Design review of the part built by this model. Coordinates are the model's own, in mm. A direction names the side the tool comes from. Coordinates: 2 decimals unless noted, no trailing zeros. Order: outer loops, then holes, each group sorted by start corner. A loop starts at its lowest first (then second) coordinate and runs counter-clockwise, first axis right, second up. Notation, with made-up numbers: M 80.5,42.5 L 124.5,42.5 A8 cw 124.5,52.5 Z; hole C 0.5,13.5 d6. An arc over 180 degrees is marked long. Answer in a Markdown table with one row per item.
from build123d import *

# Parameters (mm, degrees)
SKETCH_1_R          = 3
SKETCH_1_R_2        = 1.55
EXTRUDE_1_DEPTH     = 30
CUT_EXTRUDE_1_DEPTH = 33.5


with BuildPart() as part:
    # 草图1 → 凸台-拉伸1 (new body)
    with BuildSketch(Plane.XY):
        Polygon((15, 0), (15, 12.5), (0, 12.5), (-15, 12.5), (-15, -24), (15, -24), align=None)
        Circle(SKETCH_1_R, mode=Mode.SUBTRACT)
        with Locations((0, 7)):
            Circle(SKETCH_1_R_2, mode=Mode.SUBTRACT)
        with Locations((7, 0)):
            Circle(SKETCH_1_R_2, mode=Mode.SUBTRACT)
        with Locations((0, -7)):
            Circle(SKETCH_1_R_2, mode=Mode.SUBTRACT)
        with Locations((-7, 0)):
            Circle(SKETCH_1_R_2, mode=Mode.SUBTRACT)
    extrude(amount=EXTRUDE_1_DEPTH)

    # 草图2 → 切除-拉伸1 (cut)
    with BuildSketch(Plane(origin=(0, 12.5, 0), x_dir=(1, 0, 0), z_dir=(0, 1, 0))):
        Polygon((-11.4, -15), (-11.4, -3.6), (0, -3.6), (11.4, -3.6), (11.4, -26.4), (0, -26.4), (-11.4, -26.4), align=None)
    extrude(amount=-CUT_EXTRUDE_1_DEPTH, mode=Mode.SUBTRACT)


solid = part.part
(1) For faces 4 (the cylindrical face through (5.77, -0.94, 28.17)), 5 (the flat face through (0, -4, 3.6)), list the 3-axis set-ups (+Z, -Z, +X, -X, +Y, -Y) from which the entire face can be reached by the end or side of a thin tool; tool diameter is ignored.
Return value:
| item | result |
|---|---|
| face 4 | +Z, -Z |
| face 5 | +Y |
(2) For line 1 along Y through (x, z) = (0, 28.1); line 2 along Z through (x, y) = (9, -18.5); line 3 along Y through (x, z) = (7, 2.5), list the stretches that pass through material, from the lowest coordinate up. Write a range as from..to.
Return value:
| item | result |
|---|---|
| line 1 | y = -24..-8.55, -5.45..-3, 3..5.45, 8.55..12.5 |
| line 2 | z = 0..3.6, 26.4..30 |
| line 3 | y = -24..-1.55, 1.55..12.5 |
(3) Insertion check: pin 1 Ø5.5 at (x, y) = (0, 0) entering from +Z; pin 2 Ø3 at (x, z) = (0, 8) entering from +Y. Each pin has a flat end and moves straight along its axis. Give the tip position at first contact, or say it passes through.
Return value:
| item | result |
|---|---|
| pin 1 | passes through |
| pin 2 | stops at y = -21 |
(4) Add section B-B, the plane x = 7. Give the boundary of the cut face in (y, z), and give its area (3 significant figures).
Return value:
| item | result |
|---|---|
| outline | M -24,0 L -1.55,0 L -1.55,3.6 L -21,3.6 L -21,26.4 L -1.55,26.4 L -1.55,30 L -24,30 Z; M 1.55,0 L 12.5,0 L 12.5,3.6 L 1.55,3.6 Z; M 1.55,26.4 L 12.5,26.4 L 12.5,30 L 1.55,30 Z |
| area | 309 mm2 |
(5) Add section C-C, the plane y = 0. Give the number of separate pieces and of enclosed holes in the cut face, and give its area (3 significant figures).
Return value:
| item | result |
|---|---|
| separate pieces | 6 |
| enclosed holes | 0 |
| area | 292 mm2 |
(6) Add section A-A, the plane y = 7. Give the boundary of the cut face in (x, z), and give its area (3 significant figures).
Return value:
| item | result |
|---|---|
| outline | M -15,0 L -1.55,0 L -1.55,3.6 L -11.4,3.6 L -11.4,26.4 L -1.55,26.4 L -1.55,30 L -15,30 Z; M 1.55,0 L 15,0 L 15,30 L 1.55,30 L 1.55,26.4 L 11.4,26.4 L 11.4,3.6 L 1.55,3.6 Z |
| area | 358 mm2 |
(7) Draft analysis for pull direction Z (two halves, no side actions). For faces 1 (the cylindrical face through (0.715, 5.625, 1.775)), 2 (the flat face through (-4, -5, 30)), 3 (the flat face through (0, -21, 15)), state which applies: pulls with the +Z half, pulls with the -Z half, needs draft (parallel to the pull), parting line crosses it, or undercut.
Return value:
| item | result |
|---|---|
| face 1 | needs draft |
| face 2 | pulls with the +Z half |
| face 3 | undercut |
